Design review of the part shown in the three views and the two pictorial views. Dimensions are in mm from the part's minimum x, y and z. Give positions to 0.01 mm unless a question says otherwise; leave off trailing zeros. Loops run counter-clockwise (first coordinate to the right, second up) from the corner with the lowest first, then second, coordinate; pieces in that order, holes last. Notation, with made-up numbers: (47, 1.5) -> (74, 1.5) arc R31 cw to (74, 40.5) -> close; hole circle Ø10 at (-35, 56). An arc over 180 degrees is marked (long way). Use CSV: the item, a comma, the result in double quotes. Start each with the question number.
Item 1: Clearance check with a flat-ended pin moving along its axis: pin 1 (1.5 mm diameter, centred on x = 24, y = 21, fed in from -Z). State where the tip first meets the part, or that it passes through.
Item 2: Wall thickness on line 1 along Y through (x, z) = (11, 0.6); line 2 along Y through (x, z) = (10.5, 0.1); line 3 along X through (y, z) = (19.25, 0.2): over which ranges is each line inside the solid? List them lowest first. Write a range as from..to.
Item 3: We need section A-A (x = 41). State the section outline as (y, z) points, plus the area to 3 significant figures.
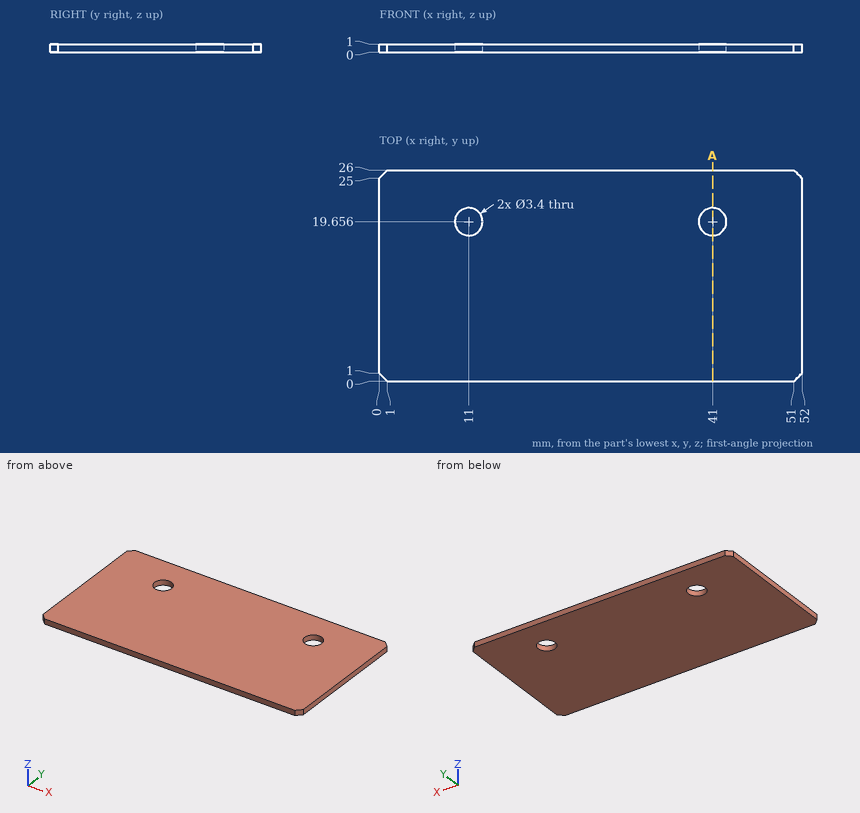
Results found:
1,pin 1,"z = 0"
2,line 1,"0..17.96, 21.36..26"
2,line 2,"0..18.03, 21.28..26"
2,line 3,"0..9.35, 12.65..39.35, 42.65..52"
3,outline,"(0, 0) -> (17.96, 0) -> (17.96, 1) -> (0, 1) -> close; (21.36, 0) -> (26, 0) -> (26, 1) -> (21.36, 1) -> close"
3,area,"22.6 mm²"
